Autodesk Inventor part; units mm, degrees
ref_plane "YZ Plane" through (0, 0, 0) normal (1, 0, 0) x (0, 1, 0)
ref_plane "XZ Plane" through (0, 0, 0) normal (0, 1, 0) x (-1, 0, 0)
ref_plane "XY Plane" through (0, 0, 0) normal (0, 0, 1) x (1, 0, 0)
sketch "スケッチ1" plane through (0, 0, 0) normal (0, 1, 0) x (-1, 0, 0)
  line L0 (0, 0) -> (30, 0)
  line L1 (30, 0) -> (30, -130)
  line L2 (30, -130) -> (0, -130)
  line L3 (0, -130) -> (0, 0)
  dimension "d0" = 30
  dimension "d1" = 130
extrude "押し出し1" add sketch "スケッチ1" along normal blind 60
sketch "スケッチ2" plane through (0, 60, 0) normal (0, 1, 0) x (1, 0, 0)
  line L0 (-30, 0) -> (0, 0)
  line L1 (0, 0) -> (-15, 0)
  line L2 (-15, 0) -> (-15, 30)
  line L3 (-15, 30) -> (0, 30)
  line L4 (0, 30) -> (0, 0)
  line L5 (0, 130) -> (-30, 130)
  line L6 (0, 130) -> (-15, 130)
  line L7 (-15, 130) -> (-15, 100)
  line L8 (-15, 100) -> (0, 100)
  line L9 (0, 100) -> (0, 130)
  dimension "d4" = 15
  dimension "d5" = 30
  dimension "d6" = 15
  dimension "d7" = 30
extrude "押し出し2" cut sketch "スケッチ2" against normal blind 60
sketch "スケッチ4" plane through (0, 0, -30) normal (1, 0, 0) x (0, 0, -1)
  line L0 (0, 0) -> (70, 0)
  line L1 (70, 60) -> (70, 0)
  line L2 (0, 0) -> (70, 0)
  line L3 (70, 0) -> (70, 60)
  line L4 (70, 60) -> (0, 60)
  line L5 (0, 60) -> (0, 0)
  point P0 (-30, 0)
extrude "押し出し3" add sketch "スケッチ4" along normal blind 15
sketch "スケッチ5" plane through (-15, 0, -30) normal (0, 0, 1) x (1, 0, 0)
  line L0 (30, 0) -> (0, 0)
  line L1 (9.0427, 0) -> (3.8663, 19.3185)
  line L2 (9.0427, 0) -> (29.0427, 0) construction
  line L3 (3.8663, 19.3185) -> (30, 26.321)
  line L4 (30, 26.321) -> (30, 0)
  line L5 (30, 0) -> (9.0427, 0)
  point P0 (15, 0)
  dimension "d15" = 20
  dimension "d16" = 105
extrude "押し出し4" cut sketch "スケッチ5" against normal blind 45.2
sketch "スケッチ6" plane through (-15, 0, -30) normal (0, 0, 1) x (1, 0, 0)
  line L0 (9.0427, 0) -> (3.8663, 19.3185)
  line L1 (3.8663, 19.3185) -> (9.0427, 0)
  line L2 (0, 0) -> (30, 0)
  line L3 (9.0427, 0) -> (30, 0)
  line L4 (30, 26.321) -> (30, 0)
  line L5 (30, 0) -> (30, 26.321)
  line L6 (30, 26.321) -> (3.8663, 19.3185)
  point P0 (15, 0)
extrude "押し出し5" add sketch "スケッチ6" against normal blind 24.8
sketch "スケッチ7" plane through (-15, 0, -30) normal (0, 0, 1) x (1, 0, 0)
  point P0 (15, 0)
sketch "スケッチ8" plane through (-15, 0, -75.2) normal (0, 0, 1) x (1, 0, 0)
  line L0 (9.0427, 0) -> (3.8663, 19.3185)
  line L1 (3.8663, 19.3185) -> (30, 26.321)
  circle A0 centre (15.5961, 14.1793) radius 1.6
  circle A1 centre (17.6666, 6.4519) radius 1.6
  point P0 (15, 0)
  dimension "d21" = 10
  dimension "d22" = 8
  dimension "d23" = 10
  dimension "d24" = 16
  dimension "d25" = 3.2
  dimension "d26" = 3.2
extrude "押し出し6" cut sketch "スケッチ8" along normal mid plane 100
sketch "スケッチ9" plane through (-15, 60, 0) normal (1, 0, 0) x (0, 0, -1)
  line L0 (0, 0) -> (30, 0)
  line L1 (0, -60) -> (0, 0)
  line L2 (100, 0) -> (130, 0)
  line L3 (130, 0) -> (130, -60)
  point P0 (15, -15)
  point P1 (15, -45)
  point P2 (115, -15)
  point P3 (115, -45)
  dimension "d29" = 15
  dimension "d30" = 15
  dimension "d31" = 15
  dimension "d32" = 45
  dimension "d33" = 15
  dimension "d34" = 15
  dimension "d35" = 30
  dimension "d36" = 15
hole "穴1" at (-15, 45, -15) at (-15, 15, -15) at (-15, 45, -115) at (-15, 15, -115) direction (-1, 0, 0) diameter 3.2 end through all
properties part number "ハンド_簡易4"
Can you work these out from the model? Positions are in its coordinate system, mm. A direction names the side the tool comes from. Give positions to 0.01 mm unless a question says otherwise; leave off trailing zeros. Loops run counter-clockwise (first coordinate to the right, second up) from the corner with the lowest first, then second, coordinate; pieces in that order, holes last. Notation, with made-up numbers: M -7,11 L 21,11 A21 cw 21,47 Z; hole C 6,60.5 d3. An arc over 180 degrees is marked long. One line per item, written item: value.
(1) Suppose I cut it at A-A on z = -115. List the corners of the cut face in (x, y) for me.
Returned:
outline: M -30,0 L -15,0 L -15,13.4 L -30,13.4 Z; M -30,16.6 L -15,16.6 L -15,43.4 L -30,43.4 Z; M -30,46.6 L -15,46.6 L -15,60 L -30,60 Z
(2) Suppose I cut it at B-B on y = 45. List the corners of the cut face in (x, z) for me, plus the area to 3 significant figures.
Returned:
outline: M -30,-130 L -15,-130 L -15,-116.6 L -30,-116.6 Z; M -30,-113.4 L -15,-113.4 L -15,-100 L 15,-100 L 15,-30 L -15,-30 L -15,-16.6 L -30,-16.6 Z; M -30,-13.4 L -15,-13.4 L -15,0 L -30,0 Z
area: 3,950 mm^2
(3) Suppose I cut it at C-C on x = -9. List the corners of the cut face in (y, z) for me.
Returned:
outline: M 0,-100 L 60,-100 L 60,-30 L 0,-30 Z; hole M 11.36,-75.2 L 19.89,-75.2 L 19.89,-54.8 L 11.36,-54.8 Z
(4) Suppose I cut it at D-D on y = 22. List the corners of the cut face in (x, z) for me.
Returned:
outline: M -30,-130 L -15,-130 L -15,-100 L 15,-100 L 15,-75.2 L -1.13,-75.2 L -1.13,-54.8 L 15,-54.8 L 15,-30 L -15,-30 L -15,0 L -30,0 Z
(5) Which directions (+Z, -Z, +X, -X, +Y, -Y) give clear straight access to the entire face, cutting with the end or side of a thin tool? Please do faces 1 (the face through (5, 13, -75.2)), 2 (the face through (-15, 30, -15)), 3 (the face through (0, 30, -100)).
Returned:
face 1: +X
face 2: +Z, +X, +Y, -Y
face 3: -Z, +X, +Y, -Y
(6) We'd pull the mould along X, two halves only. Please class faces 4 (the face through (-30, 30, -64)), 5 (the face through (-15, 30, -115)), 6 (the face through (1.07, 6.52, -87.43)): released by +X, released by -X, zero draft, split by the parting line, or undercut.
Returned:
face 4: released by -X
face 5: released by +X
face 6: undercut
(7) I need wall thicknesses on line 1 (Y direction, x = -19, z = -115); line 2 (Z direction, x = -20, y = 45); line 3 (Z direction, x = -9, y = 13). Which ranges of each line are inside material? Lowest first, please.
Returned:
line 1: 0 to 13.4, 16.6 to 43.4, 46.6 to 60
line 2: -130 to -116.6, -113.4 to -16.6, -13.4 to 0
line 3: -100 to -75.2, -54.8 to -30
(8) Will these pins go through, and if not, where does the flat tip stop? pin 1 (1.9 mm diameter, centred on y = 15, z = -115, fed in from +X); pin 2 (9 mm diameter, centred on x = 1, y = 23.5, fed in from -Z); pin 3 (3 mm diameter, centred on x = -17.5, y = 45.5, fed in from +Z); pin 4 (9 mm diameter, centred on y = 22.5, z = -10.5, fed in from +X).
Returned:
pin 1: through
pin 2: z = -100
pin 3: z = 0
pin 4: x = -15
